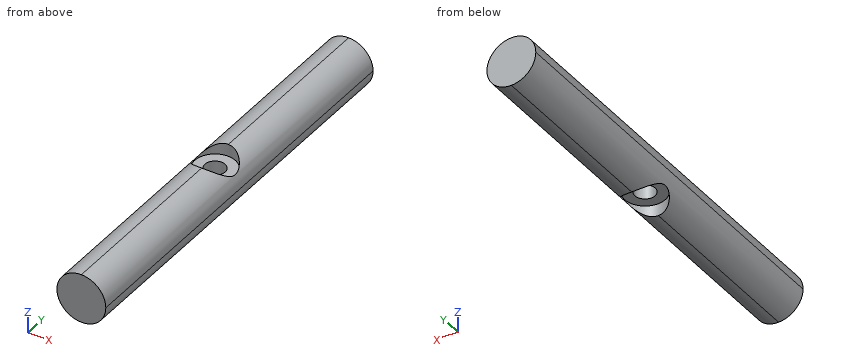
```python
from build123d import *

# Parameters (mm, degrees)
SKETCH1_W           = 12
SKETCH1_H           = 12
BOSS_EXTRUDE1_DEPTH = 100
CUT_EXTRUDE1_REACH  = 103.43
SKETCH5_R           = 2.5
SKETCH6_R           = 5
CUT_EXTRUDE3_DEPTH  = 3
CUT_EXTRUDE4_START  = -3
SKETCH7_R           = 5
SKETCH7_R_2         = 2.5
CUT_EXTRUDE4_DEPTH  = 3
CUT_EXTRUDE5_DEPTH  = 100


with BuildPart() as part:
    # Sketch1 → Boss-Extrude1 (new body)
    with BuildSketch(Plane(origin=(0, 0, 0), x_dir=(1, 0, 0), z_dir=(0, 1, 0))):
        with Locations((6, -6)):
            Rectangle(SKETCH1_W, SKETCH1_H)
    extrude(amount=BOSS_EXTRUDE1_DEPTH)

    # Sketch5 → Cut-Extrude1 (cut, up to next)
    with BuildSketch(Plane.XY.offset(12), mode=Mode.PRIVATE) as cut_extrude1_sk1:
        with Locations((6, 50)):
            Circle(SKETCH5_R)
    cut_extrude1_tool1 = extrude(cut_extrude1_sk1.sketch, amount=-CUT_EXTRUDE1_REACH, mode=Mode.PRIVATE) & part.part
    add(cut_extrude1_tool1.solids().sort_by_distance((6, 50, 12))[0], mode=Mode.SUBTRACT)

    # Sketch6 → Cut-Extrude3 (cut)
    with BuildSketch(Plane.XY.offset(12)):
        with Locations((6, 50)):
            Circle(SKETCH6_R)
    extrude(amount=-CUT_EXTRUDE3_DEPTH, mode=Mode.SUBTRACT)

    # Sketch7 → Cut-Extrude4 (cut)
    with BuildSketch(Plane(origin=(0, 0, 0), x_dir=(-1, 0, 0), z_dir=(0, 0, -1)).offset(CUT_EXTRUDE4_START)):
        with Locations(Location((-6, 50, 0), (0, 0, 180))):
            Circle(SKETCH7_R)
        with Locations(Location((-6, 50, 0), (0, 0, 180))):
            Circle(SKETCH7_R_2, mode=Mode.SUBTRACT)
    extrude(amount=CUT_EXTRUDE4_DEPTH, mode=Mode.SUBTRACT)

    # Sketch8 → Cut-Extrude5 (cut)
    with BuildSketch(Plane(origin=(0, 100, 0), x_dir=(1, 0, 0), z_dir=(0, 1, 0))):
        with BuildLine():
            Line((0, -12), (6, -12))
            ThreePointArc((6, -12), (1.757359303, -10.242640677), (0, -5.999999971))
            Line((0, -5.999999971), (0, -12))
        make_face()
        with BuildLine():
            Line((12, -12), (12, -6))
            ThreePointArc((12, -6), (10.242640687, -10.242640687), (6, -12))
            Line((6, -12), (12, -12))
        make_face()
        with BuildLine():
            ThreePointArc((5.999999987, 0), (10.242640683, -1.757359308), (12, -6))
            Line((12, -6), (12, 0))
            Line((12, 0), (5.999999987, 0))
        make_face()
        with BuildLine():
            ThreePointArc((0, -5.999999971), (1.757359319, -1.757359307), (5.999999987, 0))
            Line((5.999999987, 0), (0, 0))
            Line((0, 0), (0, -5.999999971))
        make_face()
    extrude(amount=-CUT_EXTRUDE5_DEPTH, mode=Mode.SUBTRACT)


solid = part.part
```
The listing builds one solid part. Answer for the finished solid, in the listing's coordinates (mm). Coordinates: 2 decimals unless noted, no trailing zeros. Write each loop counter-clockwise with the first axis right and the second up, starting at its lowest first coordinate (ties: lowest second). Pieces come first, ordered by that corner, then holes. Notation, with made-up numbers: (81.25, 59) - (125.25, 59) arc R34 ccw to (125.25, 94) - close; hole circle Ø6 at (3, 75.5). An arc over 180 degrees is marked (long way). Return JSON: item names as keys, results as strings. Group by question number.
1. Given pin 1 (1.5 mm diameter, centred on y = 75, z = 8, fed in from -X); pin 2 (3 mm diameter, centred on x = 8.5, y = 82, fed in from -Z); pin 3 (2 mm diameter, centred on x = 11, y = 38, fed in from -Z); pin 4 (3 mm diameter, centred on x = 6, y = 50, fed in from -Z) (1 decimal), each flat-ended and moving along its own axis, determine where each tip first touches the part or whether it passes through.
2. A cutting plane is placed at B-B, the plane x = 4.75. Determine the outline of the cut face in (y, z).
3. Straight lines are drawn through the part: L1, parallel to Y at x = 6, z = 10.3; L2, parallel to X at y = 54, z = 2.25; L3, parallel to Y at x = 4.5, z = 3.5. For each, find the intervals that lie inside material, in ascending order.
4. A cutting plane is placed at C-C, the plane y = 50. Determine the outline of the cut face in (x, z).
5. A cutting plane is placed at A-A, the plane z = 10.75. Determine the outline of the cut face in (x, y), plus the area to 3 significant figures.
6. A cutting plane is placed at D-D, the plane y = 34. Determine the outline of the cut face in (x, z), plus the area to 3 significant figures.
Ans:
{
 "1": {"pin 1": "x = 0.13", "pin 2": "z = 0.08", "pin 3": "z = 1.53", "pin 4": "through"},
 "2": {"outline": "(0, 0.13) - (45.16, 0.13) - (45.16, 3) - (47.83, 3) - (47.83, 9) - (45.16, 9) - (45.16, 11.87) - (0, 11.87) - close; (52.17, 3) - (54.84, 3) - (54.84, 0.13) - (100, 0.13) - (100, 11.87) - (54.84, 11.87) - (54.84, 9) - (52.17, 9) - close"},
 "3": {"L1": "0 to 45, 55 to 100", "L2": "1.32 to 3, 9 to 10.68", "L3": "0 to 48, 52 to 100"},
 "4": {"outline": "(1, 2.68) - (1, 3) - (3.5, 3) - (3.5, 9) - (1, 9) - (1, 9.32) arc R6 ccw to start; (8.5, 3) - (11, 3) - (11, 2.68) arc R6 ccw to (11, 9.32) - (11, 9) - (8.5, 9) - close"},
 "5": {"outline": "(2.33, 0) - (9.67, 0) - (9.67, 46.6) arc R5 cw to (2.33, 46.6) - close; (2.33, 53.4) arc R5 cw to (9.67, 53.4) - (9.67, 100) - (2.33, 100) - close", "area": "667 mm²"},
 "6": {"outline": "circle Ø12 at (6, 6)", "area": "113 mm²"}
}
